Model file for the job. Use its own axes, mm. A direction names the side the tool comes from. Coordinates: 2 decimals unless noted, no trailing zeros. Write each loop counter-clockwise with the first axis right and the second up, starting at its lowest first coordinate (ties: lowest second). Pieces come first, ordered by that corner, then holes. Notation, with made-up numbers: M 76,83 L 99,83 A25 cw 99,115 Z; hole C 11,86.25 d4. An arc over 180 degrees is marked long. One line per question, with ' | ' between items. Start each with the question number.
(1) Flat gauge pin, fed straight in: pin 1 Ø0.5 at (x, y) = (-0.5, 0.5) entering from +Z. Where does the tip first touch, or does it go through?
(2) Tool access for faces 1 (the face through (2, 1, 0)), 2 (the face through (5.5, 1, -7)), 3 (the face through (-0.5, 1, -7)): list every direction of +Z, -Z, +X, -X, +Y, -Y with a clear straight run to the whole face (end or side of a thin tool).
(3) Wall check: probe 1 along X at (y, z) = (1.45, -16.5); probe 2 along Z at (x, y) = (2.5, 0.7); probe 3 along X at (y, z) = (1.5, -3). Give the ranges that are in metal, low to high.
(4) Cut at B-B (z = -17.5). Write the cut outline in (x, y).
(5) Cut at A-A (x = 3.5). Write the cut outline in (y, z), plus the area to 3 significant figures.
(6) Cut at D-D (z = -6.5). Write the cut outline in (x, y), plus the area to 3 significant figures.
(7) Cut at C-C (y = 1.55). Write the cut outline in (x, z).
(8) Two-plate mould, pull along X, no slides. Class faces 4 (the face through (0, 1, -3)), 5 (the face through (3, 2, -10)), 6 (the face through (3.172, 1.014, -17.554)): +X half, -X half, draft (parallel to the pull), parting line (faces both ways), or undercut.
Autodesk Inventor part; units mm, degrees
ref_plane "YZ Plane" through (0, 0, 0) normal (1, 0, 0) x (0, 1, 0)
ref_plane "XZ Plane" through (0, 0, 0) normal (0, 1, 0) x (-1, 0, 0)
ref_plane "XY Plane" through (0, 0, 0) normal (0, 0, 1) x (1, 0, 0)
sketch "Sketch3" plane through (0, 0, 0) normal (0, 1, 0) x (-1, 0, 0)
  line L0 (0, 0) -> (-5, 0)
  line L1 (-5, 0) -> (-5, -7)
  line L2 (0, 0) -> (0, -7)
  line L3 (0, -7) -> (1, -7)
  line L4 (1, -7) -> (1, -20)
  line L5 (-5, -7) -> (-6, -7)
  line L6 (-6, -7) -> (-6, -20)
  line L7 (-6, -20) -> (1, -20)
  dimension "d9" = 5
  dimension "d10" = 7
  dimension "d11" = 1
  dimension "d12" = 13
  dimension "d13" = 1
extrude "Extrusion3" add sketch "Sketch3" along normal blind 2
sketch "Sketch4" plane through (0, 2, 0) normal (0, 1, 0) x (1, 0, 0)
  line L0 (-1, 20) -> (-1, 7)
  line L1 (-1, 20) -> (2.5, 20)
  line L2 (6, 20) -> (-1, 20)
  line L3 (2.5, 20) -> (2.5, 16.5)
  circle A0 centre (2.5, 16.5) radius 1.25
  point P0 (0, 0)
  dimension "d16" = 3.5
  dimension "d17" = 3.5
  dimension "d18" = 2.5
extrude "Extrusion4" cut sketch "Sketch4" against normal blind 2
properties part number "HINGE B"
Filled in:
1) pin 1: z = -7
2) face 1: +Z, +X, -X, +Y, -Y | face 2: +Z, +X, +Y, -Y | face 3: +Z, -X, +Y, -Y
3) probe 1: -1 to 1.25, 3.75 to 6 | probe 2: -20 to -17.75, -15.25 to 0 | probe 3: 0 to 5
4) outline: M -1,0 L 1.75,0 L 1.75,2 L -1,2 Z; M 3.25,0 L 6,0 L 6,2 L 3.25,2 Z
5) outline: M 0,-20 L 2,-20 L 2,-17.25 L 0,-17.25 Z; M 0,-15.75 L 2,-15.75 L 2,0 L 0,0 Z | area: 37.0 mm²
6) outline: M 0,0 L 5,0 L 5,2 L 0,2 Z | area: 10.0 mm²
7) outline: M -1,-20 L 6,-20 L 6,-7 L 5,-7 L 5,0 L 0,0 L 0,-7 L -1,-7 Z; hole C 2.5,-16.5 d2.5
8) face 4: -X half | face 5: draft | face 6: undercut
